The model under review builds one solid part; all positions refer to its coordinate system, in mm. A direction names the side the tool comes from. Coordinates: 2 decimals unless noted, no trailing zeros. Loops run counter-clockwise (first coordinate to the right, second up) from the corner with the lowest first, then second, coordinate; pieces in that order, holes last. Notation, with made-up numbers: M -30,42 L 27,42 A11 ccw 27,56 Z; hole C 6,-22.75 d1. An arc over 180 degrees is marked long. Use one line per item in the form item = value.
```python
from build123d import *

# Parameters (mm, degrees)
F1_DEPTH = 0.4


with BuildPart() as f1:
    # F0 (on Top) → F1 (new body)
    with BuildSketch(Plane.XY):
        with BuildLine():
            Line((134.117601, 52.35192), (104.790399, 52.35192))
            ThreePointArc((104.790399, 52.35192), (98.599906, 50.364955), (94.722175, 45.146388))
            Line((94.722175, 45.146388), (90.439587, 53.731151))
            Line((90.439587, 53.731151), (78.773495, 30.448411))
            Line((78.773495, 30.448411), (78.773495, 52.493423))
            ThreePointArc((78.773495, 52.493423), (72.923348, 51.04402), (68.176621, 47.33005))
            Line((68.176621, 47.33005), (55.041848, 31.619177))
            Line((55.041848, 31.619177), (41.907075, 47.33005))
            ThreePointArc((41.907075, 47.33005), (37.160347, 51.04402), (31.3102, 52.493423))
            Line((31.3102, 52.493423), (31.3102, 15.584978))
            ThreePointArc((31.3102, 15.584978), (34.975357, 7.386031), (43.52908, 4.649262))
            Line((43.52908, 4.649262), (43.52908, 26.505338))
            Line((43.52908, 26.505338), (55.041848, 12.091459))
            Line((55.041848, 12.091459), (66.554615, 26.505338))
            Line((66.554615, 26.505338), (66.554615, 4.581898))
            Line((66.554615, 4.581898), (83.704581, 4.581914))
            ThreePointArc((83.704581, 4.581914), (91.70244, 8.42165), (93.707784, 17.063867))
            Line((93.707784, 17.063867), (86.238848, 17.063867))
            Line((86.238848, 17.063867), (90.309106, 25.609449))
            Line((90.309106, 25.609449), (98.430799, 9.756892))
            ThreePointArc((98.430799, 9.756892), (112.588106, 3.440158), (121.785738, 15.919502))
            Line((121.785738, 15.919502), (121.785738, 39.959846))
            Line((121.785738, 39.959846), (127.466301, 39.959846))
            ThreePointArc((127.466301, 39.959846), (129.789281, 40.322243), (131.891491, 41.374992))
            Line((131.891491, 41.374992), (131.891491, 15.021686))
            ThreePointArc((131.891491, 15.021686), (134.662869, 7.916194), (141.513281, 4.563521))
            Line((141.513281, 4.563521), (149.037555, 4.563528))
            ThreePointArc((149.037555, 4.563528), (157.035414, 8.403264), (159.040758, 17.045482))
            Line((159.040758, 17.045482), (151.571822, 17.045482))
            Line((151.571822, 17.045482), (155.64208, 25.591063))
            Line((155.64208, 25.591063), (163.763773, 9.738506))
            ThreePointArc((163.763773, 9.738506), (167.159763, 6.0203), (171.974498, 4.545128))
            Line((171.974498, 4.545128), (178.360625, 4.545128))
            Line((178.360625, 4.545128), (186.306138, 4.545128))
            ThreePointArc((186.306138, 4.545128), (201.425191, 19.664181), (186.306138, 34.783235))
            Line((186.306138, 34.783235), (176.385451, 34.783235))
            ThreePointArc((176.385451, 34.783235), (173.751636, 37.41705), (176.385451, 40.050866))
            Line((176.385451, 40.050866), (186.306138, 40.050866))
            ThreePointArc((186.306138, 40.050866), (194.459994, 43.760102), (197.021679, 52.3439))
            Line((197.021679, 52.3439), (176.385451, 52.3439))
            ThreePointArc((176.385451, 52.3439), (167.316213, 49.307242), (161.90404, 41.421765))
            Line((161.90404, 41.421765), (155.772561, 53.712765))
            Line((155.772561, 53.712765), (144.402741, 31.021313))
            Line((144.402741, 31.021313), (144.402741, 41.55154))
            ThreePointArc((144.402741, 41.55154), (141.420105, 49.008622), (134.117601, 52.35192))
        make_face()
        Polygon((110.209341, 39.95985), (110.209341, 14.101218), (97.309523, 39.95985), align=None, mode=Mode.SUBTRACT)
        with BuildLine():
            Line((32.510204, 15.584978), (32.510204, 51.195543))
            ThreePointArc((32.510204, 51.195543), (37.18689, 49.67996), (40.986429, 46.560362))
            Line((40.986429, 46.560362), (55.041848, 29.748278))
            Line((55.041848, 29.748278), (69.097267, 46.560362))
            ThreePointArc((69.097267, 46.560362), (72.896805, 49.67996), (77.573491, 51.195543))
            Line((77.573491, 51.195543), (77.573491, 25.374748))
            Line((77.573491, 25.374748), (90.437222, 51.04769))
            Line((90.437222, 51.04769), (95.369863, 41.15985))
            Line((95.369863, 41.15985), (111.409341, 9.007538))
            Line((111.409341, 9.007538), (111.409341, 41.15985))
            Line((111.409341, 41.15985), (96.710893, 41.15985))
            Line((96.710893, 41.15985), (95.529365, 43.528313))
            ThreePointArc((95.529365, 43.528313), (98.792773, 49.000858), (104.790399, 51.151916))
            Line((104.790399, 51.151916), (134.087416, 51.151916))
            ThreePointArc((134.087416, 51.151916), (140.560905, 48.17076), (143.202737, 41.55154))
            Line((143.202737, 41.55154), (143.202737, 25.947649))
            Line((143.202737, 25.947649), (155.770196, 51.029305))
            Line((155.770196, 51.029305), (162.525616, 37.48757))
            Line((162.525616, 37.48757), (168.213113, 26.086565))
            Line((168.213113, 26.086565), (173.694601, 15.098518))
            Line((173.694601, 15.098518), (186.306138, 15.098518))
            ThreePointArc((186.306138, 15.098518), (190.467475, 19.259855), (186.306138, 23.421193))
            Line((186.306138, 23.421193), (176.385451, 23.421193))
            ThreePointArc((176.385451, 23.421193), (173.177011, 23.797627), (170.142836, 24.906486))
            Line((170.142836, 24.906486), (162.743499, 39.739006))
            ThreePointArc((162.743499, 39.739006), (167.494805, 47.917086), (176.385451, 51.143896))
            Line((176.385451, 51.143896), (195.918921, 51.143896))
            ThreePointArc((195.918921, 51.143896), (193.203195, 44.16594), (186.306138, 41.25087))
            Line((186.306138, 41.25087), (176.385451, 41.25087))
            ThreePointArc((176.385451, 41.25087), (172.551632, 37.41705), (176.385451, 33.583231))
            Line((176.385451, 33.583231), (186.306138, 33.583231))
            ThreePointArc((186.306138, 33.583231), (200.225188, 19.664181), (186.306138, 5.745132))
            Line((186.306138, 5.745132), (178.360625, 5.745132))
            Line((178.360625, 5.745132), (171.993494, 5.745132))
            ThreePointArc((171.993494, 5.745132), (167.793729, 7.039214), (164.831771, 10.28567))
            Line((164.831771, 10.28567), (155.602871, 28.29936))
            Line((155.602871, 28.29936), (149.671091, 15.845478))
            Line((149.671091, 15.845478), (158.027767, 15.845478))
            ThreePointArc((158.027767, 15.845478), (155.791616, 8.790163), (149.037554, 5.763532))
            Line((149.037554, 5.763532), (141.564783, 5.763525))
            ThreePointArc((141.564783, 5.763525), (135.529592, 8.746533), (133.091494, 15.021686))
            Line((133.091494, 15.021686), (133.091494, 44.478871))
            ThreePointArc((133.091494, 44.478871), (130.731983, 42.051456), (127.466301, 41.15985))
            Line((127.466301, 41.15985), (120.585735, 41.15985))
            Line((120.585735, 41.15985), (120.585735, 15.893338))
            ThreePointArc((120.585735, 15.893338), (112.293961, 4.603626), (99.498797, 10.304056))
            Line((99.498797, 10.304056), (90.269897, 28.317746))
            Line((90.269897, 28.317746), (84.338117, 15.863864))
            Line((84.338117, 15.863864), (92.694793, 15.863864))
            ThreePointArc((92.694793, 15.863864), (90.458642, 8.808548), (83.70458, 5.781918))
            Line((83.70458, 5.781918), (67.786207, 5.781903))
            ThreePointArc((67.786207, 5.781903), (67.771236, 5.78189), (67.756265, 5.7819))
            ThreePointArc((67.756265, 5.7819), (67.755442, 5.781902), (67.754619, 5.781903))
            Line((67.754619, 5.781903), (67.754619, 29.930541))
            Line((67.754619, 29.930541), (55.041848, 14.014268))
            Line((55.041848, 14.014268), (42.329077, 29.930541))
            Line((42.329077, 29.930541), (42.329077, 5.781903))
            ThreePointArc((42.329077, 5.781903), (35.387045, 8.647569), (32.510204, 15.584978))
        make_face(mode=Mode.SUBTRACT)
        with BuildLine():
            Line((174.437, 16.298518), (170.982292, 23.223732))
            ThreePointArc((170.982292, 23.223732), (173.637761, 22.473948), (176.385451, 22.221193))
            Line((176.385451, 22.221193), (186.306138, 22.221193))
            ThreePointArc((186.306138, 22.221193), (189.267475, 19.259855), (186.306138, 16.298518))
            Line((186.306138, 16.298518), (174.437, 16.298518))
        make_face(mode=Mode.SUBTRACT)
    extrude(amount=F1_DEPTH)


solid = f1.part
```
1. Insertion check: P1, Ø5, axis at x = 103.5, y = 42.5, coming from the -Z side. The pin has a flat end and moves straight along its axis. Give the tip position at first contact, or say it passes through.
Response values:
P1 = 0
2. Wall thickness on line 1 along Y through (x, z) = (182.5, 0.2); line 2 along Y through (x, z) = (189.5, 0.2); line 3 along Y through (x, z) = (100.5, 0.25): over which ranges is each line inside the solid? List them lowest first. Write a range as from..to.
Response values:
line_1 = 4.55..5.75, 15.1..16.3, 22.22..23.42, 33.58..34.78, 40.05..41.25, 51.14..52.34
line_2 = 4.89..6.12, 16.59..21.93, 33.21..34.44, 40.53..41.8, 51.14..52.34
line_3 = 6.85..8.7, 30.88..33.56, 39.96..41.16, 50.12..51.45
3. Add section B-B (z = 0.3). Count the separate pieces of the cut face and the enclosed holes in it, then the cut area to 3 significant figures.
Response values:
separate_pieces = 1
enclosed_holes = 3
area = 1,110 mm^2
4. Add section D-D (x = 81). State the section outline as (y, z) points.
Response values:
outline = M 4.58,0 L 5.78,0 L 5.78,0.4 L 4.58,0.4 Z; M 32.21,0 L 34.89,0 L 34.89,0.4 L 32.21,0.4 Z
5. The part is to be moulded in two halves that separate along Y. For faces 4 (the face through (158.88, 47.48, 0.2)), 5 (the face through (87.346, 22.178, 0.197)), 6 (the face through (34.88, 7.47, 0.2)), 7 (the face through (155.86, 8.87, 0.2)), say which applies: pulls with the +Y half, pulls with the -Y half, needs draft (parallel to the pull), parting line crosses it, or undercut.
Response values:
face_4 = pulls with the +Y half
face_5 = undercut
face_6 = pulls with the -Y half
face_7 = undercut
6. Machinability: for faces 1 (the face through (194.37, 43.66, 0.2)), 2 (the face through (189.267, 19.325, 0.197)), 3 (the face through (48.57, 39.36, 0.2)), which of the approach directions +Z, -Z, +X, -X, +Y, -Y give a long, thin tool a straight path to every point of the face, cutting with its end or side? Answer none if there is none.
Response values:
face_1 = +Z, -Z, +X
face_2 = +Z, -Z
face_3 = +Z, -Z, +Y
7. Add section A-A (x = 59.5). State the section outline as (y, z) points.
Response values:
outline = M 17.67,0 L 19.6,0 L 19.6,0.4 L 17.67,0.4 Z; M 35.08,0 L 36.95,0 L 36.95,0.4 L 35.08,0.4 Z
